from build123d import *

# Parameters (mm, degrees)
EXTRUDE1_DEPTH          = 54.5
CUT_EXTRUDE1_DEPTH      = 55.854885702
CUT_EXTRUDE1_DEPTH_BACK = 55.854885702
SKETCH2_R               = 1.5
CUT_EXTRUDE2_DEPTH      = 55.854885702
CUT_EXTRUDE2_DEPTH_BACK = 55.854885702


with BuildPart() as part:
    # Sketch1 → Extrude1 (new, symmetric)
    with BuildSketch(Plane(origin=(0, 0, 0), x_dir=(0, 0, -1), z_dir=(1, 0, 0))):
        with BuildLine():
            Line((-1.715977045, 5), (1.715977045, 5))
            ThreePointArc((1.715977045, 5), (2.824752941, 4.540729986), (3.284022955, 3.43195409))
            Line((3.284022955, 3.43195409), (3.284022955, -3.43195409))
            ThreePointArc((3.284022955, -3.43195409), (2.824752941, -4.540729986), (1.715977045, -5))
            Line((1.715977045, -5), (-1.715977045, -5))
            ThreePointArc((-1.715977045, -5), (-2.672673527, -4.674330771), (-3.23197526, -3.832600305))
            ThreePointArc((-3.23197526, -3.832600305), (-3.383560587, -3.204564402), (-3.507961213, -2.570583572))
            ThreePointArc((-3.507961213, -2.570583572), (-3.356955711, -1.900195953), (-3.674237451, -1.290643232))
            ThreePointArc((-3.674237451, -1.290643232), (-3.698584955, -0.968220458), (-3.715977045, -0.645347786))
            ThreePointArc((-3.715977045, -0.645347786), (-3.479865934, 0), (-3.715977045, 0.645347786))
            ThreePointArc((-3.715977045, 0.645347786), (-3.698584955, 0.968220458), (-3.674237451, 1.290643232))
            ThreePointArc((-3.674237451, 1.290643232), (-3.356955711, 1.900195953), (-3.507961213, 2.570583572))
            ThreePointArc((-3.507961213, 2.570583572), (-3.383560587, 3.204564402), (-3.23197526, 3.832600305))
            ThreePointArc((-3.23197526, 3.832600305), (-2.672673527, 4.674330771), (-1.715977045, 5))
        make_face()
        with BuildLine():
            Line((-1.715977045, 4), (1.715977045, 4))
            ThreePointArc((1.715977045, 4), (2.11764616, 3.833623205), (2.284022955, 3.43195409))
            Line((2.284022955, 3.43195409), (2.284022955, -3.43195409))
            ThreePointArc((2.284022955, -3.43195409), (2.11764616, -3.833623205), (1.715977045, -4))
            Line((1.715977045, -4), (-1.715977045, -4))
            ThreePointArc((-1.715977045, -4), (-2.062553328, -3.882021902), (-2.265167971, -3.577093618))
            ThreePointArc((-2.265167971, -3.577093618), (-2.729865934, 0), (-2.265167971, 3.577093618))
            ThreePointArc((-2.265167971, 3.577093618), (-2.062553328, 3.882021902), (-1.715977045, 4))
        make_face(mode=Mode.SUBTRACT)
    extrude(amount=EXTRUDE1_DEPTH, both=True)

    # Sketch2 → Cut-Extrude1 (cut, two sides: drawn at the far end of the back side and taken through both)
    with BuildSketch(Plane(origin=(0, 0, 0), x_dir=(1, 0, 0), z_dir=(0, 1, 0)).offset(-CUT_EXTRUDE1_DEPTH_BACK)):
        with Locations(Location((-51.25, 0, 0), (0, 0, 270))):
            Circle(SKETCH2_R)
        with Locations(Location((51.25, 0, 0), (0, 0, 90))):
            Circle(SKETCH2_R)
    extrude(amount=CUT_EXTRUDE1_DEPTH + CUT_EXTRUDE1_DEPTH_BACK, mode=Mode.SUBTRACT)

    # Sketch3 → Cut-Extrude2 (cut, two sides: drawn at the far end of the back side and taken through both)
    with BuildSketch(Plane(origin=(0, 0, 0), x_dir=(0, 0, -1), z_dir=(1, 0, 0)).offset(-CUT_EXTRUDE2_DEPTH_BACK)):
        Polygon((0, -1.75), (0, 1.75), (3.034022955, 1.75), (3.034022955, 3), (4.284022955, 3), (4.284022955, -3), (3.034022955, -3), (3.034022955, -1.75), align=None)
    extrude(amount=CUT_EXTRUDE2_DEPTH + CUT_EXTRUDE2_DEPTH_BACK, mode=Mode.SUBTRACT)


solid = part.part
Could you check a few things on this model? Use its own coordinates, in mm. A direction names the side the tool comes from. Coordinates: 2 decimals unless noted, no trailing zeros. Order: outer loops, then holes, each group sorted by start corner. A loop starts at its lowest first (then second) coordinate and runs counter-clockwise, first axis right, second up. Notation, with made-up numbers: (43, 16.25) - (77, 16.25) arc R22 ccw to (77, 26.25) - close; hole circle Ø5 at (9.5, 76). An arc over 180 degrees is marked (long way). Answer in a Markdown table with one row per item. Add a question column.
(1) If we mould it in two halves opening along Z, with no side actions, what happens to faces 1 (the face through (-52.714, -4.507, -0.325)), 2 (the face through (1, 5, 0))? For each: released by +Z, released by -Z, zero draft, split by the parting line, or undercut.
(2) On a 3-axis mill with a long thin cutter (end or side, diameter ignored), from which of +Z, -Z, +X, -X, +Y, -Y can I reach the whole of each face in a straight line? I mean faces 3 (the face through (52.714, -4.507, 0.325)), 4 (the face through (1, 3, -2.284)). Say none if no direction works.
(3) I need wall thicknesses on L1, parallel to X at y = 4.4, z = 0; L2, parallel to Y at x = -25, z = 1; L3, parallel to Z at x = -51.25, y = -4.45. Which ranges of each line are inside material? Lowest first, please.
(4) If we section it at C-C, the plane x = -51.25: State how many separate pieces and enclosed holes the cut face has, then the cut area to 3 significant figures.
(5) If we section it at A-A, the plane z = 0: Please give me the cut outline in (x, y), then the cut area to 3 significant figures.
(6) Will these pins go through, and if not, where does the flat tip stop? pin 1 (1.8 mm diameter, centred on x = 51.25, z = 0, fed in from +Y); pin 2 (1.3 mm diameter, centred on x = -18.5, y = -2.5, fed in from +Z); pin 3 (0.8 mm diameter, centred on x = 27, z = -2.5, fed in from -Y).
Results are:
| question | item | result |
|---|---|---|
| 1 | face 1 | undercut |
| 1 | face 2 | zero draft |
| 2 | face 3 | +Y, -Y |
| 2 | face 4 | +X, -X |
| 3 | L1 | x = -54.5 to -52.75, -49.75 to 49.75, 52.75 to 54.5 |
| 3 | L2 | y = -5 to -4, 4 to 5 |
| 3 | L3 | z = -2.91 to -1.5, 1.5 to 2.91 |
| 4 | separate pieces | 3 |
| 4 | enclosed holes | 0 |
| 4 | area | 16.6 mm2 |
| 5 | outline | (-54.5, -5) - (-52.75, -5) - (-52.75, -4) - (-54.5, -4) - close; (-54.5, 4) - (-52.75, 4) - (-52.75, 5) - (-54.5, 5) - close; (-49.75, -5) - (49.75, -5) - (49.75, -4) - (-49.75, -4) - close; (-49.75, 4) - (49.75, 4) - (49.75, 5) - (-49.75, 5) - close; (52.75, -5) - (54.5, -5) - (54.5, -4) - (52.75, -4) - close; (52.75, 4) - (54.5, 4) - (54.5, 5) - (52.75, 5) - close |
| 5 | area | 206 mm2 |
| 6 | pin 1 | passes through |
| 6 | pin 2 | stops at z = 3.51 |
| 6 | pin 3 | stops at y = -4.95 |
